from build123d import *

# Parameters (mm, degrees)
SKETCH002_R        = 12
PAD002_DEPTH       = 14
CHAMFER_SIZE       = 0.6
POCKET_DEPTH       = 73.431239
POCKET_DEPTH_BACK  = 87.431239
POLARPATTERN_COUNT = 12
SKETCH_R           = 3.5
POCKET001_DEPTH    = 2
SKETCH004_R        = 2.9
POCKET002_DEPTH    = 9
SKETCH005_W        = 0.7
SKETCH005_H        = 6.120777
PAD_DEPTH          = 3


with BuildPart() as part:
    # Sketch002 → Pad002 (new body)
    with BuildSketch(Plane.XY):
        Circle(SKETCH002_R)
    extrude(amount=PAD002_DEPTH)

    # Chamfer
    chamfer_edges = [part.edges().sort_by_distance(p)[0] for p in [
        (-12, 0, 14),
        (-12, 0, 0),
    ]]
    chamfer(chamfer_edges, length=CHAMFER_SIZE)

    # Sketch003 → Pocket (cut, two sides)
    with BuildSketch(Plane.XY) as pocket_sk:
        Polygon((-1.058613, 12.1), (-0.944878, 10.8), (0.944878, 10.8), (1.058613, 12.1), align=None)
    pocket = extrude(amount=-POCKET_DEPTH, mode=Mode.SUBTRACT) + extrude(pocket_sk.sketch, amount=POCKET_DEPTH_BACK, mode=Mode.SUBTRACT)

    # PolarPattern: Pocket ×12 about axis
    polarpattern_axis = Axis((0, 0, 0), (0, 0, 1))
    for i in range(1, POLARPATTERN_COUNT):
        add(pocket.rotate(polarpattern_axis, i * 360 / POLARPATTERN_COUNT), mode=Mode.SUBTRACT)

    # Sketch → Pocket001 (cut)
    with BuildSketch(Plane.XY):
        Circle(SKETCH_R)
    extrude(amount=POCKET001_DEPTH, mode=Mode.SUBTRACT)

    # Sketch004 → Pocket002 (cut)
    with BuildSketch(Plane.XY):
        Circle(SKETCH004_R)
    extrude(amount=POCKET002_DEPTH, mode=Mode.SUBTRACT)

    # Sketch005 (on Face78 of Pocket002) → Pad (join)
    with BuildSketch(Plane(origin=(0, 0, 9), x_dir=(1, 0, 0), z_dir=(0, 0, -1))):
        with Locations((0, 0.049592)):
            Rectangle(SKETCH005_W, SKETCH005_H)
    extrude(amount=PAD_DEPTH)


solid = part.part
Geometry: final body of the model. Coordinates: model frame, mm. A direction names the side the tool comes from. Round coordinates to 2 decimals unless told otherwise and drop trailing zeros. Order: outer loops, then holes, each group sorted by start corner. A loop starts at its lowest first (then second) coordinate and runs counter-clockwise, first axis right, second up. Notation, with made-up numbers: (28, 43.25) - (55, 43.25) arc R26 cw to (55, 60.25) - close; hole circle Ø4 at (31, 87.25). An arc over 180 degrees is marked (long way). Write each question's results on one line, items separated by ' | '.
Item 1: Mould query, pull axis X, two halves, no side actions, for faces 5 (the flat face through (9.36, -5.39, 7.1)), 6 (the conical face through (2.999, -11.305, 0.296)), 7 (the conical face through (-11.305, -2.999, 0.296)). Classes: pulls with the +X half, pulls with the -X half, needs draft (parallel to the pull), parting line crosses it, or undercut.
Completed:
face 5: undercut | face 6: pulls with the +X half | face 7: pulls with the -X half
Item 2: Reachability of faces 1 (the flat face through (6.546, 9.349, 7.098)), 2 (the conical face through (-3.055, -11.29, 0.296)), 3 (the flat face through (10.8, 0, 7)), 4 (the flat face through (-0.35, 0, 8)) from +Z, -Z, +X, -X, +Y, -Y: full face, straight path, thin tool, end or side. Return the list, or none.
Completed:
face 1: +Z, -Z, +Y | face 2: -Z, -X, -Y | face 3: +Z, -Z, +X | face 4: -Z
Item 3: Material intervals for line 1 along Y through (x, z) = (0, 0.7); line 2 along X through (y, z) = (9.25, 1); line 3 along X through (y, z) = (0, 4), sorted ascending. Write a range as [from, to].
Completed:
line 1: [-10.8, -3.5], [3.5, 10.8] | line 2: [-7.64, -6.48], [-5.58, 5.58], [6.48, 7.64] | line 3: [-10.8, -2.9], [2.9, 10.8]
Item 4: Section A-A, the plane x = 0. Return the cut outline in (y, z).
Completed:
outline: (-10.8, 0) - (-3.5, 0) - (-3.5, 2) - (-2.9, 2) - (-2.9, 6) - (2.9, 6) - (2.9, 2) - (3.5, 2) - (3.5, 0) - (10.8, 0) - (10.8, 14) - (-10.8, 14) - close
Item 5: First-contact query: pin 1 Ø3.5 at (x, y) = (-1.5, -0.5) entering from -Z; pin 2 Ø1.5 at (x, z) = (0, 3.5) entering from -Y; pin 3 Ø4 at (x, y) = (0, 0) entering from -Z. Flat tips, straight axial feed; report the tip coordinate or a pass-through.
Completed:
pin 1: z = 2 | pin 2: y = -10.8 | pin 3: z = 6
Item 6: Section B-B, the plane y = 0. Return the cut outline in (x, z).
Completed:
outline: (-10.8, 0) - (-3.5, 0) - (-3.5, 2) - (-2.9, 2) - (-2.9, 9) - (-0.35, 9) - (-0.35, 6) - (0.35, 6) - (0.35, 9) - (2.9, 9) - (2.9, 2) - (3.5, 2) - (3.5, 0) - (10.8, 0) - (10.8, 14) - (-10.8, 14) - close
